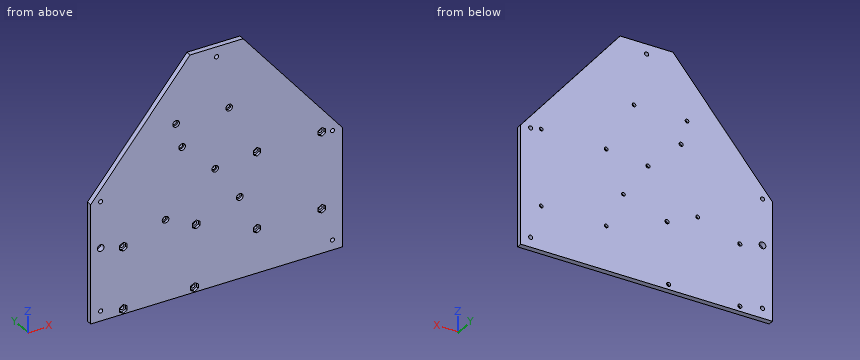
Autodesk Inventor part; units mm, degrees
ref_plane "YZ Plane" through (0, 0, 0) normal (1, 0, 0) x (0, 1, 0)
ref_plane "XZ Plane" through (0, 0, 0) normal (0, 1, 0) x (-1, 0, 0)
ref_plane "XY Plane" through (0, 0, 0) normal (0, 0, 1) x (1, 0, 0)
sketch "Sketch1" plane through (0, 0, 0) normal (0, 1, 0) x (-1, 0, 0)
  line L0 (0, 0) -> (-190, 0)
  line L1 (-95, 180) -> (-75, 180)
  line L2 (-75, 180) -> (0, 90)
  line L3 (-95, 180) -> (-115, 180)
  line L4 (-115, 180) -> (-190, 90)
  line L5 (0, 0) -> (0, 90)
  line L6 (-190, 0) -> (-190, 90)
  dimension "d1" = 190
  dimension "d39" = 20
  dimension "d40" = 20
extrude "Extrusion1" add sketch "Sketch1" along normal blind 4
sketch "Sketch14" plane through (0, 4, 0) normal (0, 1, 0) x (1, 0, 0)
  line L0 (190, 0) -> (0, 0)
  line L1 (0, 0) -> (0, -7.5)
  line L2 (0, 0) -> (0, -15)
  line L3 (0, -90) -> (75, -180)
  circle A0 centre (7.5, -7.5) radius 1.55
  circle A1 centre (7.5, -90) radius 1.55
  line L4 (75, -180) -> (115, -180)
  circle A2 centre (182.5, -7.5) radius 1.55
  circle A3 centre (182.5, -90) radius 1.55
  circle A4 centre (95, -172.5) radius 1.55
  dimension "d68" = 7.5
  dimension "d71" = 3.1
  dimension "d72" = 3.1
  dimension "d74" = 3.1
extrude "Extrusion10" cut sketch "Sketch14" against normal blind 10
sketch "Sketch17" plane through (0, 4, 0) normal (0, 1, 0) x (1, 0, 0)
  line L0 (93.28, -54.34) -> (12, -54.34)
  line L1 (12, -54.34) -> (12, -1)
  line L2 (12, -1) -> (93.28, -1)
  line L3 (93.28, -1) -> (93.28, -54.34)
  line L4 (93.28, -54.34) -> (93.28, -50.7586)
  circle A0 centre (79.5513, -50.7586) radius 1.55
  circle A1 centre (24.6238, -50.7586) radius 1.55
  line L5 (93.28, -1) -> (93.28, -3.8194)
  circle A2 centre (78.3321, -3.8194) radius 1.55
  circle A3 centre (24.6238, -3.8194) radius 1.55
  point P0 (0, 0)
  dimension "d101" = 81.28
  dimension "d102" = 53.34
  dimension "d106" = 3.1
  dimension "d107" = 3.1
  dimension "d111" = 3.1
  dimension "d112" = 3.1
  dimension "d113" = 14.9479
  dimension "d114" = 2.8194
  dimension "d115" = 12.6238
  dimension "d116" = 2.8194
  dimension "d117" = 12.6238
  dimension "d118" = 3.5814
  dimension "d119" = 3.5814
  dimension "d120" = 13.7287
sketch "Sketch18" plane through (0, 4, 0) normal (0, 1, 0) x (1, 0, 0)
  line L0 (190, 0) -> (0, 0)
  line L1 (190, -90) -> (190, 0)
  line L2 (175, -10) -> (125, -10)
  line L3 (122, -13) -> (122, -92)
  line L4 (125, -95) -> (175, -95)
  line L5 (178, -92) -> (178, -13)
  circle A0 centre (174.5, -91.5) radius 1.375
  circle A1 centre (125.5, -91.5) radius 1.4481
  circle A2 centre (125.5, -33.5) radius 1.375
  circle A3 centre (174.5, -33.5) radius 1.375
  arc A4 (125, -10) -> (122, -13) centre (125, -13) ccw
  arc A5 (178, -13) -> (175, -10) centre (175, -13) ccw
  arc A6 (175, -95) -> (178, -92) centre (175, -92) ccw
  arc A7 (122, -92) -> (125, -95) centre (125, -92) ccw
  point P0 (122, -10)
  dimension "d129" = 2.75
  dimension "d130" = 3.5
  dimension "d131" = 3.5
  dimension "d132" = 49
  dimension "d133" = 3.5
  dimension "d134" = 2.75
  dimension "d135" = 3.5
  dimension "d136" = 58
  dimension "d137" = 2.75
  dimension "d138" = 3.5
  dimension "d139" = 49
  dimension "d140" = 3
  dimension "d141" = 3
  dimension "d142" = 3
  dimension "d143" = 3
sketch "Sketch19" plane through (0, 4, 0) normal (0, 1, 0) x (1, 0, 0)
  line L0 (49.4722, -56.3802) -> (119.4722, -56.3802)
  line L1 (119.4722, -56.3802) -> (119.4722, -154.8802)
  line L2 (119.4722, -154.8802) -> (49.4722, -154.8802)
  line L3 (49.4722, -154.8802) -> (49.4722, -56.3802)
  circle A0 centre (56.4722, -61.3802) radius 1.375
  circle A1 centre (112.4722, -61.3802) radius 1.375
  circle A2 centre (104.4722, -131.2502) radius 1.375
  circle A3 centre (64.4722, -131.2502) radius 1.375
  point P0 (0, 0)
  dimension "d144" = 70
  dimension "d145" = 98.5
  dimension "d151" = 2.75
  dimension "d152" = 2.75
  dimension "d153" = 2.75
  dimension "d154" = 2.75
  dimension "d155" = 5
  dimension "d156" = 69.87
  dimension "d157" = 5
  dimension "d158" = 69.87
  dimension "d159" = 40
  dimension "d160" = 56
extrude "Extrusion13" cut sketch "Sketch17" against normal through all contours A0 | A1 | A2 | A3
extrude "Extrusion14" cut sketch "Sketch18" against normal through all contours A0 | A1 | A2 | A3
extrude "Extrusion15" cut sketch "Sketch19" against normal through all contours A0 | A1 | A2 | A3
sketch "Sketch22" plane through (0, 0, 0) normal (0, -1, 0) x (1, 0, 0)
  circle A0 centre (112.4722, 61.3802) radius 1.375
  circle A1 centre (112.4722, 61.3802) radius 2.5
  circle A2 centre (56.4722, 61.3802) radius 1.375
  circle A3 centre (56.4722, 61.3802) radius 2.5
  circle A4 centre (64.4722, 131.2502) radius 1.375
  circle A5 centre (64.4722, 131.2502) radius 2.5
  circle A6 centre (104.4722, 131.2502) radius 1.375
  circle A7 centre (104.4722, 131.2502) radius 2.5
  point P0 (0, 0)
  dimension "d171" = 5
  dimension "d172" = 5
  dimension "d173" = 5
  dimension "d174" = 5
extrude "Extrusion16" cut sketch "Sketch22" against normal blind 2
sketch "Sketch23" plane through (0, 0, 0) normal (0, -1, 0) x (1, 0, 0)
  circle A0 centre (125.5, 33.5) radius 1.375
  circle A1 centre (125.5, 91.5) radius 1.4481
  circle A2 centre (174.5, 91.5) radius 1.375
  circle A3 centre (174.5, 33.5) radius 1.375
  line L0 (174.5, 30.3) -> (171.7287, 31.9)
  line L1 (171.7287, 31.9) -> (171.7287, 35.1)
  line L2 (171.7287, 35.1) -> (174.5, 36.7)
  line L3 (174.5, 36.7) -> (177.2713, 35.1)
  line L4 (177.2713, 35.1) -> (177.2713, 31.9)
  line L5 (177.2713, 31.9) -> (174.5, 30.3)
  line L6 (125.5, 30.3) -> (122.7287, 31.9)
  line L7 (122.7287, 31.9) -> (122.7287, 35.1)
  line L8 (122.7287, 35.1) -> (125.5, 36.7)
  line L9 (125.5, 36.7) -> (128.2713, 35.1)
  line L10 (128.2713, 35.1) -> (128.2713, 31.9)
  line L11 (128.2713, 31.9) -> (125.5, 30.3)
  line L12 (125.5, 88.3) -> (122.7287, 89.9)
  line L13 (122.7287, 89.9) -> (122.7287, 93.1)
  line L14 (122.7287, 93.1) -> (125.5, 94.7)
  line L15 (125.5, 94.7) -> (128.2713, 93.1)
  line L16 (128.2713, 93.1) -> (128.2713, 89.9)
  line L17 (128.2713, 89.9) -> (125.5, 88.3)
  line L18 (174.5, 88.3) -> (171.7287, 89.9)
  line L19 (171.7287, 89.9) -> (171.7287, 93.1)
  line L20 (171.7287, 93.1) -> (174.5, 94.7)
  line L21 (174.5, 94.7) -> (177.2713, 93.1)
  line L22 (177.2713, 93.1) -> (177.2713, 89.9)
  line L23 (177.2713, 89.9) -> (174.5, 88.3)
  circle A4 centre (78.3321, 3.8194) radius 1.55
  circle A5 centre (79.5513, 50.7586) radius 1.55
  circle A6 centre (24.6238, 50.7586) radius 1.55
  circle A7 centre (24.6238, 3.8194) radius 1.55
  line L24 (78.3321, 0.5194) -> (75.4742, 2.1694)
  line L25 (75.4742, 2.1694) -> (75.4742, 5.4694)
  line L26 (75.4742, 5.4694) -> (78.3321, 7.1194)
  line L27 (78.3321, 7.1194) -> (81.19, 5.4694)
  line L28 (81.19, 5.4694) -> (81.19, 2.1694)
  line L29 (81.19, 2.1694) -> (78.3321, 0.5194)
  line L30 (24.6238, 0.5194) -> (21.7659, 2.1694)
  line L31 (21.7659, 2.1694) -> (21.7659, 5.4694)
  line L32 (21.7659, 5.4694) -> (24.6238, 7.1194)
  line L33 (24.6238, 7.1194) -> (27.4817, 5.4694)
  line L34 (27.4817, 5.4694) -> (27.4817, 2.1694)
  line L35 (27.4817, 2.1694) -> (24.6238, 0.5194)
  line L36 (79.5513, 47.4586) -> (76.6934, 49.1086)
  line L37 (76.6934, 49.1086) -> (76.6934, 52.4086)
  line L38 (76.6934, 52.4086) -> (79.5513, 54.0586)
  line L39 (79.5513, 54.0586) -> (82.4092, 52.4086)
  line L40 (82.4092, 52.4086) -> (82.4092, 49.1086)
  line L41 (82.4092, 49.1086) -> (79.5513, 47.4586)
  line L42 (24.6238, 47.4586) -> (21.7659, 49.1086)
  line L43 (21.7659, 49.1086) -> (21.7659, 52.4086)
  line L44 (21.7659, 52.4086) -> (24.6238, 54.0586)
  line L45 (24.6238, 54.0586) -> (27.4817, 52.4086)
  line L46 (27.4817, 52.4086) -> (27.4817, 49.1086)
  line L47 (27.4817, 49.1086) -> (24.6238, 47.4586)
  point P0 (0, 0)
extrude "Extrusion17" cut sketch "Sketch23" against normal blind 2 contours A0 | A1 | A2 | A3 | L0 L1 L2 L3 L4 L5 | L6 L7 L8 L9 L10 L11 | L12 L13 L14 L15 L16 L17 | L18 L19 L20 L21 L22 L23 | A4 | A5 | L24 L25 L26 L27 L28 L29 | L30 L31 L32 L33 L34 L35 | L36 L37 L38 L39 L40 L41 | L42 L43 L44 L45 L46 L47
sketch "Sketch24" plane through (0, 4, 0) normal (0, 1, 0) x (1, 0, 0)
  circle A0 centre (56.4722, -61.3802) radius 2.5
  circle A1 centre (93.9722, -88.3552) radius 1.55
  circle A2 centre (68.9722, -112.4052) radius 1.55
  point P0 (0, 0)
  dimension "d206" = 3.1
  dimension "d208" = 3.1
  dimension "d209" = 25
  dimension "d210" = 24.05
extrude "Extrusion18" cut sketch "Sketch24" against normal blind 10 contours A1 | A2
sketch "Sketch25" plane through (0, 4, 0) normal (0, 1, 0) x (1, 0, 0)
  circle A0 centre (7.5, -90) radius 1.55
  circle A1 centre (7.5, -55) radius 2.5
  point P0 (0, 0)
  dimension "d202" = 5
extrude "Extrusion19" cut sketch "Sketch25" against normal blind 10 contours A1
sketch "Sketch26" plane through (0, 0, 0) normal (0, -1, 0) x (1, 0, 0)
  circle A0 centre (93.9722, 88.3552) radius 1.55
  circle A1 centre (93.9722, 88.3552) radius 2.5
  circle A2 centre (68.9722, 112.4052) radius 1.55
  circle A3 centre (68.9722, 112.4052) radius 2.5
  point P0 (0, 0)
  dimension "d211" = 5
  dimension "d212" = 5
extrude "Extrusion20" cut sketch "Sketch26" against normal blind 2
properties part number "bp_v2" material "PET Plastic"
Verification items for the finished model (mm, model axes). Round coordinates to 2 decimals unless told otherwise and drop trailing zeros. Order: outer loops, then holes, each group sorted by start corner. A loop starts at its lowest first (then second) coordinate and runs counter-clockwise, first axis right, second up. Notation, with made-up numbers: (36.25, 60) -> (48.25, 60) arc R18 ccw to (48.25, 93) -> close; hole circle Ø6 at (48, 45.5). An arc over 180 degrees is marked (long way). Put each result on its own line as item: value.
1) Section check B-B (y = 3.2). Give the number of separate pieces and of enclosed holes in the cut face, then the cut area to 3 significant figures.
Final values:
separate pieces: 1
enclosed holes: 20
area: 27,300 mm^2
2) Depth check by flat-ended pin: pin 1 (1 mm diameter, centred on y = 1, z = 91, fed in from +X); pin 2 (2.5 mm diameter, centred on x = 174.5, z = 33.5, fed in from -Y); pin 3 (0.6 mm diameter, centred on y = 1, z = 91, fed in from +X); pin 4 (3 mm diameter, centred on x = 173.5, z = 34, fed in from -Y). Enter the tip coordinate at first touch or a pass-through.
Final values:
pin 1: stops at x = 189.58
pin 2: passes through
pin 3: stops at x = 189.42
pin 4: stops at y = 2
3) Material ranges on line 1 (X direction, y = 1.9, z = 92.5); line 2 (X direction, y = 3.25, z = 49.5); line 3 (Z direction, x = 174.5, y = 3.4) (3 decimals), recorded low to high.
Final values:
line 1: x = 2.08 to 122.73, 128.27 to 171.73, 177.27 to 187.92
line 2: x = 0 to 23.72, 25.53 to 78.65, 80.46 to 190
line 3: z = 0 to 32.125, 34.875 to 90.125, 92.875 to 108.6
4) Section check C-C (z = 117). Record the cut outline in (x, y), then the cut area to 3 significant figures.
Final values:
outline: (22.5, 0) -> (167.5, 0) -> (167.5, 4) -> (22.5, 4) -> close
area: 580 mm^2
5) Section check A-A (x = 47). Record the cut outline in (y, z).
Final values:
outline: (0, 0) -> (4, 0) -> (4, 146.4) -> (0, 146.4) -> close
